```python
from build123d import *

# Parameters (mm, degrees)
SKETCH1_W               = 70
SKETCH1_H               = 70
SKETCH1_W_2             = 50
SKETCH1_H_2             = 50
BOSS_EXTRUDE1_DEPTH     = 60
SKETCH2_W               = 60
SKETCH2_H               = 50
BOSS_EXTRUDE2_DEPTH     = 300
SKETCH3_R               = 15
BOSS_EXTRUDE3_DEPTH     = 25
SKETCH4_R               = 10
CUT_EXTRUDE1_DEPTH      = 56
SKETCH5_R               = 10
CUT_EXTRUDE2_DEPTH      = 6
CUT_EXTRUDE2_DEPTH_BACK = 56
CUT_EXTRUDE3_START      = -20
SKETCH8_R               = 2.5
CUT_EXTRUDE3_DEPTH      = 30
SKETCH9_R               = 5
CUT_EXTRUDE4_DEPTH      = 17


with BuildPart() as part:
    # Sketch1 → Boss-Extrude1 (new body)
    with BuildSketch(Plane(origin=(0, 0, 0), x_dir=(1, 0, 0), z_dir=(0, 1, 0))):
        Rectangle(SKETCH1_W, SKETCH1_H)
        Rectangle(SKETCH1_W_2, SKETCH1_H_2, mode=Mode.SUBTRACT)
    extrude(amount=BOSS_EXTRUDE1_DEPTH)

    # Sketch2 → Boss-Extrude2 (add)
    with BuildSketch(Plane(origin=(35, 0, 0), x_dir=(0, 0, -1), z_dir=(1, 0, 0))):
        with Locations((0, 30)):
            Rectangle(SKETCH2_W, SKETCH2_H)
    extrude(amount=BOSS_EXTRUDE2_DEPTH)

    # Sketch3 → Boss-Extrude3 (add)
    with BuildSketch(Plane.ZY.offset(35)):
        with Locations((0, 30)):
            Circle(SKETCH3_R)
    extrude(amount=BOSS_EXTRUDE3_DEPTH)

    # Sketch4 → Cut-Extrude1 (cut, through all)
    with BuildSketch(Plane(origin=(0, 55, 0), x_dir=(1, 0, 0), z_dir=(0, 1, 0))):
        with Locations((285, 0)):
            Circle(SKETCH4_R)
    extrude(amount=-CUT_EXTRUDE1_DEPTH, mode=Mode.SUBTRACT)

    # Sketch5 → Cut-Extrude2 (cut, two sides)
    with BuildSketch(Plane(origin=(0, 55, 0), x_dir=(1, 0, 0), z_dir=(0, 1, 0))) as cut_extrude2_sk:
        with Locations((44, 0)):
            Circle(SKETCH5_R)
    extrude(amount=CUT_EXTRUDE2_DEPTH, mode=Mode.SUBTRACT)
    extrude(cut_extrude2_sk.sketch, amount=-CUT_EXTRUDE2_DEPTH_BACK, mode=Mode.SUBTRACT)

    # Sketch8 → Cut-Extrude3 (cut)
    with BuildSketch(Plane(origin=(0, 55, 0), x_dir=(1, 0, 0), z_dir=(0, 1, 0)).offset(CUT_EXTRUDE3_START)):
        with Locations((255.00002319, -0.037301815)):
            Circle(SKETCH8_R)
        with Locations((299.967684086, 25.999392937)):
            Circle(SKETCH8_R)
        with Locations((300.032292724, -25.962091123)):
            Circle(SKETCH8_R)
    extrude(amount=-CUT_EXTRUDE3_DEPTH, mode=Mode.SUBTRACT)

    # Sketch9 → Cut-Extrude4 (cut)
    with BuildSketch(Plane(origin=(335, 0, 0), x_dir=(0, 0, -1), z_dir=(1, 0, 0))):
        with Locations((-15.340483078, 20.605088766)):
            Circle(SKETCH9_R)
        with Locations((4.659516922, 20.605088766)):
            Circle(SKETCH9_R)
    extrude(amount=-CUT_EXTRUDE4_DEPTH, mode=Mode.SUBTRACT)


solid = part.part
```
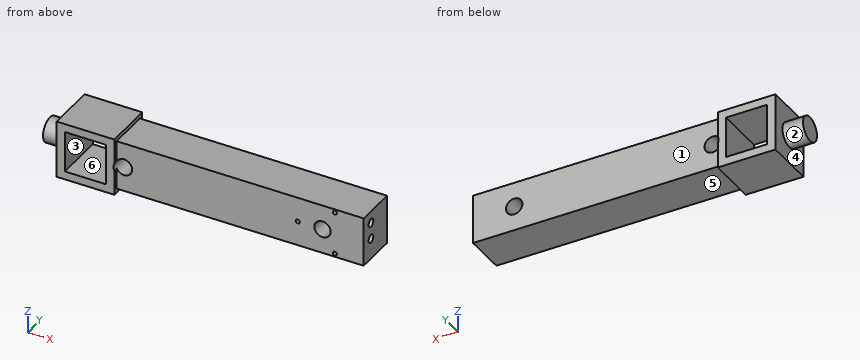
Source: CAD feature listing. Evaluate the final solid. Frame: model axes, mm. Face numbers are marked on the shaded views. A direction names the side the tool comes from. Give positions to 0.01 mm unless a question says otherwise; leave off trailing zeros. Loops run counter-clockwise (first coordinate to the right, second up) from the corner with the lowest first, then second, coordinate; pieces in that order, holes last. Notation, with made-up numbers: (31, 29.25) -> (59, 29.25) arc R21 ccw to (59, 57.25) -> close; hole circle Ø11 at (-39.75, 86). An arc over 180 degrees is marked (long way). Use a Markdown table: item, result. Add a question column.
(1) Section query B-B (y = 30). Output: boundary loops of the cut face in (x, z), then the cut area to 3 significant figures.
(2) Section query D-D (x = 138). Output: boundary loops of the cut face in (y, z).
(3) Pull-direction query (X, two-part tool) for the marked faces 4, 5 and 6; classes: +X half, -X half, draft (parallel to the pull), parting line (faces both ways), or undercut.
(4) Access query for the marked faces 1, 2 and 3. Directions: +Z, -Z, +X, -X, +Y, -Y. A direction counts if a zero-diameter tool reaches every point of the face in a straight line with its end or side. Return the directions, or none.
(5) First-contact query: pin 1 Ø15 at (x, y) = (211.5, 39) entering from -Z; pin 2 Ø4 at (x, z) = (300.03, 25.96) entering from -Y; pin 3 Ø1 at (y, z) = (50.5, -21) entering from -X. Flat tips, straight axial feed; report the tip coordinate or a pass-through.
(6) Section query A-A (x = 44). Output: boundary loops of the cut face in (y, z).
(7) Section query C-C (x = -11.5). Output: boundary loops of the cut face in (y, z).
(8) Ray query, line 1 (X direction, y = 26.5, z = -11); line 2 (Z direction, x = 285, y = 44); line 3 (X direction, y = 56, z = -1). Return the intervals inside material, ascending.
Checked values:
| question | item | result |
|---|---|---|
| 1 | outline | (-60, -15) -> (-35, -15) -> (-35, -35) -> (35, -35) -> (35, -30) -> (335, -30) -> (335, 30) -> (35, 30) -> (35, 35) -> (-35, 35) -> (-35, 15) -> (-60, 15) -> close; hole (-25, -25) -> (25, -25) -> (25, 25) -> (-25, 25) -> close; hole circle Ø20 at (44, 0); hole circle Ø5 at (255, 0.04); hole circle Ø20 at (285, 0); hole circle Ø5 at (299.97, -26); hole circle Ø5 at (300.03, 25.96) |
| 1 | area | 20,500 mm^2 |
| 2 | outline | (5, -30) -> (55, -30) -> (55, 30) -> (5, 30) -> close |
| 3 | face 4 | -X half |
| 3 | face 5 | draft |
| 3 | face 6 | undercut |
| 4 | face 1 | +Z, -Z, +X, +Y |
| 4 | face 2 | -X |
| 4 | face 3 | +Y, -Y |
| 5 | pin 1 | z = -30 |
| 5 | pin 2 | y = 35 |
| 5 | pin 3 | x = -35 |
| 6 | outline | (5, -30) -> (55, -30) -> (55, -10) -> (5, -10) -> close; (5, 10) -> (55, 10) -> (55, 30) -> (5, 30) -> close |
| 7 | outline | (0, -35) -> (60, -35) -> (60, -25) -> (0, -25) -> close; (0, 25) -> (60, 25) -> (60, 35) -> (0, 35) -> close |
| 8 | line 1 | -60 to -25, 25 to 335 |
| 8 | line 2 | -30 to -10, 10 to 30 |
| 8 | line 3 | -35 to -25, 25 to 34.05 |
